Check sheet for the modelled part. Datum: model origin and axes. Units: mm. Face numbers are marked on the shaded views. A direction names the side the tool comes from. Give positions to 0.01 mm unless a question says otherwise; leave off trailing zeros. Order: outer loops, then holes, each group sorted by start corner. A loop starts at its lowest first (then second) coordinate and runs counter-clockwise, first axis right, second up.
from build123d import *

# Parameters (mm, degrees)
SKETCH_1_W             = 94.247779608
SKETCH_1_H             = 6
EXTRUDE_1_DEPTH        = 6
EXTRUDE_2_DEPTH        = 6
PATTERN_LINEAR_1_COUNT = 20
PATTERN_LINEAR_1_PITCH = 4.71238898
SKETCH_4_W             = 27
SKETCH_4_H             = 6
SKETCH_4_R             = 1.5
EXTRUDE_1_2_DEPTH      = 6
CUT_EXTRUDE_1_DEPTH    = 10
CUT_EXTRUDE_START      = -24
CUT_EXTRUDE_2_DEPTH    = 79.74919082
FILLET_1_R             = 0.25


with BuildPart() as part:
    # 草图1 → Extrude 1 (new body)
    with BuildSketch(Plane.XY):
        with Locations((47.123889804, -3)):
            Rectangle(SKETCH_1_W, SKETCH_1_H)
    extrude(amount=EXTRUDE_1_DEPTH)

    # 草图2 → 拉伸2 (add)
    with BuildSketch(Plane.XY.offset(6)):
        Polygon((0, 0), (1.228399541, 3.375), (2.492683328, 3.375), (3.721082869, 0), align=None)
    extrude_2 = extrude(amount=-EXTRUDE_2_DEPTH)

    # 阵列(线性)1: 拉伸2 ×20
    with Locations(*[(i * PATTERN_LINEAR_1_PITCH, 0, 0) for i in range(1, PATTERN_LINEAR_1_COUNT)]):
        add(extrude_2)

    # 草图4 → Extrude 1 2 (add)
    with BuildSketch(Plane.XY.offset(6)):
        with Locations((-13.5, -3)):
            Rectangle(SKETCH_4_W, SKETCH_4_H)
        with Locations((-24, -3)):
            Circle(SKETCH_4_R, mode=Mode.SUBTRACT)
        with Locations((-16, -3)):
            Circle(SKETCH_4_R, mode=Mode.SUBTRACT)
        with Locations((-8, -3)):
            Circle(SKETCH_4_R, mode=Mode.SUBTRACT)
    extrude(amount=-EXTRUDE_1_2_DEPTH)

    # 草图5 → 切除-拉伸1 (cut)
    with BuildSketch(Plane.XY.offset(6)):
        Polygon((94.247779608, -6), (94.247779608, 6), (75.398223686, 6), (75.398223686, 0), (75.398223686, -6), align=None)
    extrude(amount=-CUT_EXTRUDE_1_DEPTH, mode=Mode.SUBTRACT)

    # 草图6 → 切除-拉伸2 (cut, through all)
    with BuildSketch(Plane.ZY.offset(27).offset(CUT_EXTRUDE_START)):
        Polygon((2.4, -5.570156212), (1.383875031, -4.3), (4.616124969, -4.3), (3.6, -5.570156212), (3.6, -6.2), (2.4, -6.2), align=None)
    extrude(amount=-CUT_EXTRUDE_2_DEPTH, mode=Mode.SUBTRACT)

    # 圆角1
    fillet_1_edges = [part.edges().sort_by_distance(p)[0] for p in [
        (36.199111843, -4.3, 1.383875031),
        (36.199111843, -4.3, 4.616124969),
    ]]
    fillet(fillet_1_edges, radius=FILLET_1_R)


solid = part.part
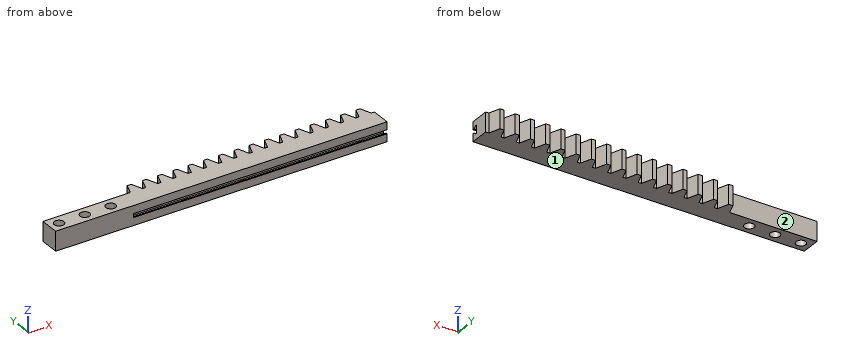
1) Depth check by flat-ended pin: pin 1 Ø0.8 at (y, z) = (-5, 2.5) entering from +X; pin 2 Ø0.5 at (x, z) = (51.5, 3) entering from +Y. Enter the tip coordinate at first touch or a pass-through.
Recorded:
pin 1: stops at x = -3
pin 2: stops at y = 0
2) Set-up check for the marked faces 1 and 2: record each of +Z, -Z, +X, -X, +Y, -Y from which the full face is reachable in a straight line by a thin tool's end or side.
Recorded:
face 1: -Z, +X, -X, +Y, -Y
face 2: +Z, -Z, -X, +Y
3) Section check B-B, the plane x = -24. Record the cut outline in (y, z).
Recorded:
outline: (-6, 0) - (-4.5, 0) - (-4.5, 6) - (-6, 6) - close; (-1.5, 0) - (0, 0) - (0, 6) - (-1.5, 6) - close
4) Material ranges on L1, parallel to Y at x = -24, z = 4; L2, parallel to X at y = -1.75, z = 0.8; L3, parallel to X at y = -3.5, z = 4.15, recorded low to high.
Recorded:
L1: y = -6 to -4.5, -1.5 to 0
L2: x = -27 to -24.83, -23.17 to -16.83, -15.17 to -8.83, -7.17 to 75.4
L3: x = -27 to -25.41, -22.59 to -17.41, -14.59 to -9.41, -6.59 to 75.4
5) Section check A-A, the plane y = -3. Record the cut outline in (x, z), then the cut area to 3 significant figures.
Recorded:
outline: (-27, 0) - (-25.5, 0) - (-25.5, 6) - (-27, 6) - close; (-22.5, 0) - (-17.5, 0) - (-17.5, 6) - (-22.5, 6) - close; (-14.5, 0) - (-9.5, 0) - (-9.5, 6) - (-14.5, 6) - close; (-6.5, 0) - (75.4, 0) - (75.4, 6) - (-6.5, 6) - close
area: 560 mm2
6) Section check C-C, the plane y = 2.5. State how many separate pieces and enclosed holes the cut face has, then the cut area to 3 significant figures.
Recorded:
separate pieces: 16
enclosed holes: 0
area: 183 mm2
